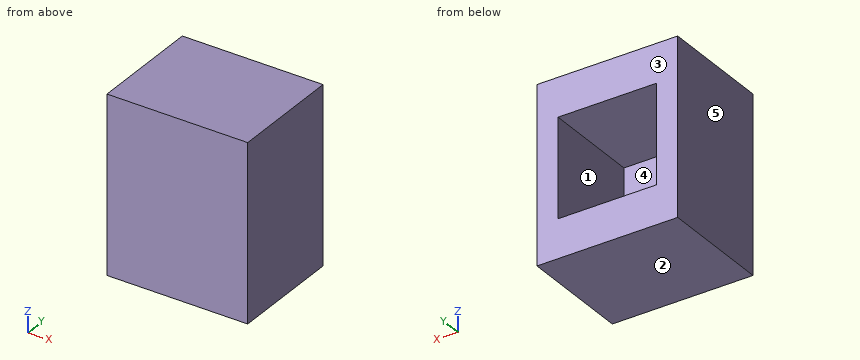
Autodesk Inventor part; units mm, degrees
ref_plane "YZ Plane" through (0, 0, 0) normal (1, 0, 0) x (0, 1, 0)
ref_plane "XZ Plane" through (0, 0, 0) normal (0, 1, 0) x (-1, 0, 0)
ref_plane "XY Plane" through (0, 0, 0) normal (0, 0, 1) x (1, 0, 0)
sketch "Sketch1" plane through (0, 0, 0) normal (0, 1, 0) x (-1, 0, 0)
  line L0 (2.5, 3.125) -> (-2.5, 3.125)
  line L1 (-2.5, 3.125) -> (-2.5, -3.125)
  line L2 (-2.5, -3.125) -> (2.5, -3.125)
  line L3 (2.5, -3.125) -> (2.5, 3.125)
  dimension "d3" = 5
extrude "Extrusion1" add sketch "Sketch1" along normal blind 4
sketch "Sketch2" plane through (0, 4, 0) normal (0, 1, 0) x (1, 0, 0)
  line L0 (-1.75, -1.75) -> (1.75, -1.75)
  line L1 (1.75, -1.75) -> (1.75, 1.75)
  line L2 (1.75, 1.75) -> (-1.75, 1.75)
  line L3 (-1.75, 1.75) -> (-1.75, -1.75)
  dimension "d9" = 3.5
extrude "Extrusion2" cut sketch "Sketch2" against normal blind 3.5
properties part number "Double Slit Centre Piece"
Read the model definition and answer for the solid it produces. Units are mm, in the model's axes. Face numbers are marked on the shaded views. A direction names the side the tool comes from. Round coordinates to 2 decimals unless told otherwise and drop trailing zeros. Loops run counter-clockwise (first coordinate to the right, second up) from the corner with the lowest first, then second, coordinate; pieces in that order, holes last. Notation, with made-up numbers: (46, -19) -> (78, -19) arc R22 cw to (78, 2) -> close; hole circle Ø9 at (-36.5, -10). An arc over 180 degrees is marked (long way). One line per item, written item: value.
1) A cutting plane is placed at C-C (x = 1.45). Determine the outline of the cut face in (y, z) (3 decimals).
Answer list:
outline: (0, -3.125) -> (4, -3.125) -> (4, -1.75) -> (0.5, -1.75) -> (0.5, 1.75) -> (4, 1.75) -> (4, 3.125) -> (0, 3.125) -> close
2) A cutting plane is placed at A-A (y = 2.75). Determine the outline of the cut face in (x, z) (3 decimals).
Answer list:
outline: (-2.5, -3.125) -> (2.5, -3.125) -> (2.5, 3.125) -> (-2.5, 3.125) -> close; hole (-1.75, -1.75) -> (1.75, -1.75) -> (1.75, 1.75) -> (-1.75, 1.75) -> close
3) A cutting plane is placed at B-B (z = 1.25). Determine the outline of the cut face in (x, y).
Answer list:
outline: (-2.5, 0) -> (2.5, 0) -> (2.5, 4) -> (1.75, 4) -> (1.75, 0.5) -> (-1.75, 0.5) -> (-1.75, 4) -> (-2.5, 4) -> close
4) A flat-ended cylindrical pin translates along its axis: P1, Ø2, axis at x = 0, z = 0, coming from the +Y side. Find the tip coordinate at first contact, or state that the pin passes through.
Answer list:
P1: stops at y = 0.5
5) Consider L1, parallel to Z at x = -0.8, y = 2.6 (3 decimals); L2, parallel to X at y = 3.65, z = 1.25; L3, parallel to Y at x = -0.4, z = -1.25. Determine where each line is inside the solid, lowest interval first. Write a range as [from, to].
Answer list:
L1: z = [-3.125, -1.75], [1.75, 3.125]
L2: x = [-2.5, -1.75], [1.75, 2.5]
L3: y = [0, 0.5]
6) For the marked faces 1 and 2, determine the directions among +Z, -Z, +X, -X, +Y, -Y from which every point of the face is accessible in a straight line to the end or side of a thin tool.
Answer list:
face 1: +Y
face 2: -Z, +X, -X, +Y, -Y
7) The mould has two halves that part along X. Classify the marked faces 3, 4 and 5: pulls with the +X half, pulls with the -X half, needs draft (parallel to the pull), parting line crosses it, or undercut.
Answer list:
face 3: needs draft
face 4: undercut
face 5: pulls with the -X half
